Source: CAD feature listing. Evaluate the final solid. Frame: model axes, mm. A direction names the side the tool comes from. Give positions to 0.01 mm unless a question says otherwise; leave off trailing zeros. Loops run counter-clockwise (first coordinate to the right, second up) from the corner with the lowest first, then second, coordinate; pieces in that order, holes last. Notation, with made-up numbers: (21.25, 86.25) -> (62.25, 86.25) arc R17 cw to (62.25, 98.25) -> close; hole circle Ø7 at (59.25, 89). An arc over 180 degrees is marked (long way). Return JSON: item names as keys, results as strings. Group by question number.
(1) Access query for faces 4 (the face through (0, 1.76, 5)), 5 (the face through (-11.79, -0.04, 5.99)). Directions: +Z, -Z, +X, -X, +Y, -Y. A direction counts if a zero-diameter tool reaches every point of the face in a straight line with its end or side. Return the directions, or none.
(2) Draft query along Z for faces 1 (the face through (16.994, -0.042, 5.235)), 2 (the face through (0, 2, 0)), 3 (the face through (7.284, 0.039, 4.595)). Return one class per face: released by +Z, released by -Z, zero draft, split by the parting line, or undercut.
(3) Cut plane C-C on z = 7. Return loops of the section in (x, y) (3 decimals), then the cut area to 3 significant figures.
(4) Ray query, line 1 (Y direction, x = 0, z = 4) (3 decimals); line 2 (Z direction, x = 11.08, y = 1.85); line 3 (X direction, y = 1.3, z = 4.66). Return the intervals inside material, ascending. Write a range as from..to.
(5) Pin query (flat end, axial travel): pin 1 (2.5 mm diameter, centred on x = -18.4, z = 4.66, fed in from +Y). Return the tip coordinate at first contact, or that it passes through.
(6) Cut plane A-A on y = 0.7. Return loops of the section in (x, z), then the cut area to 3 significant figures.
(7) Cut plane B-B on x = 11.08. Return loops of the section in (y, z) (3 decimals).
```python
from build123d import *

# Parameters (mm, degrees)
SKETCH1_W                 = 45.16
SKETCH1_H                 = 5.99
BOSS_EXTRUDE1_DEPTH       = 9.32
F_3_0MM_DOWEL_HOLE1_D     = 3
F_3_0MM_DOWEL_HOLE1_DEPTH = 10
F_3_0MM_DOWEL_HOLE1_TIP   = 0.901290929


with BuildPart() as part:
    # Sketch1 → Boss-Extrude1 (new body)
    with BuildSketch(Plane.XY):
        Rectangle(SKETCH1_W, SKETCH1_H)
        with BuildLine():
            Line((5.523637636, -1.760435864), (-5.523637636, -1.760435864))
            ThreePointArc((-5.523637636, -1.760435864), (-7.284073501, 0), (-5.523637636, 1.760435864))
            Line((-5.523637636, 1.760435864), (5.523637636, 1.760435864))
            ThreePointArc((5.523637636, 1.760435864), (7.284073501, 0), (5.523637636, -1.760435864))
        make_face(mode=Mode.SUBTRACT)
    extrude(amount=BOSS_EXTRUDE1_DEPTH)

    # Ø3.0mm Dowel Hole1
    with Locations(Plane(origin=(0, 2.995, 0), x_dir=(1, 0, 0), z_dir=(0, 1, 0))):
        with Locations((-18.4, -4.66), (-11.1, -4.66), (11.08, -4.66), (18.38, -4.66)):
            Hole(F_3_0MM_DOWEL_HOLE1_D / 2, depth=F_3_0MM_DOWEL_HOLE1_DEPTH)
            with Locations((0, 0, -(F_3_0MM_DOWEL_HOLE1_DEPTH + F_3_0MM_DOWEL_HOLE1_TIP / 2))):  # 118° drill point
                Cone(0, F_3_0MM_DOWEL_HOLE1_D / 2, F_3_0MM_DOWEL_HOLE1_TIP, mode=Mode.SUBTRACT)


solid = part.part
```
Answers:
{
 "1": {"face 4": "+Z, -Z", "face 5": "+Y, -Y"},
 "2": {"face 1": "undercut", "face 2": "released by -Z", "face 3": "zero draft"},
 "3": {"outline": "(-22.58, -2.995) -> (22.58, -2.995) -> (22.58, 2.995) -> (-22.58, 2.995) -> close; hole (-5.524, -1.76) -> (5.524, -1.76) arc R1.76 ccw to (5.524, 1.76) -> (-5.524, 1.76) arc R1.76 ccw to start", "area": "222 mm²"},
 "4": {"line 1": "-2.995..-1.76, 1.76..2.995", "line 2": "0..3.16, 6.16..9.32", "line 3": "-22.58..-19.9, -16.9..-12.6, -9.6..-6.71, 6.71..9.58, 12.58..16.88, 19.88..22.58"},
 "5": {"pin 1": "through"},
 "6": {"outline": "(-22.58, 0) -> (-7.14, 0) -> (-7.14, 9.32) -> (-22.58, 9.32) -> close; (7.14, 0) -> (22.58, 0) -> (22.58, 9.32) -> (7.14, 9.32) -> close; hole circle Ø3 at (-18.4, 4.66); hole circle Ø3 at (-11.1, 4.66); hole circle Ø3 at (11.08, 4.66); hole circle Ø3 at (18.38, 4.66)", "area": "260 mm²"},
 "7": {"outline": "(-2.995, 0) -> (2.995, 0) -> (2.995, 3.16) -> (-2.995, 3.16) -> close; (-2.995, 6.16) -> (2.995, 6.16) -> (2.995, 9.32) -> (-2.995, 9.32) -> close"}
}
